Design review of the part built by this model. Coordinates are the model's own, in mm. A direction names the side the tool comes from. Give positions to 0.01 mm unless a question says otherwise; leave off trailing zeros. Write each loop counter-clockwise with the first axis right and the second up, starting at its lowest first coordinate (ties: lowest second). Pieces come first, ordered by that corner, then holes. Notation, with made-up numbers: M -15.75,72 L 39.25,72 A24 ccw 39.25,99 Z; hole C 71,27.25 d10. An arc over 180 degrees is marked long. One line per item, written item: value. Start each with the question number.
```python
from build123d import *

# Parameters (mm, degrees)
BOSS_EXTRUDE1_DEPTH = 10
CHAMFER1_SIZE       = 0.4


with BuildPart() as part:
    # Sketch1 → Boss-Extrude1 (new body)
    with BuildSketch(Plane(origin=(0, 0, 0), x_dir=(1, 0, 0), z_dir=(0, 1, 0))):
        with BuildLine():
            Line((0, 0.4), (7, 0.4))
            ThreePointArc((7, 0.4), (7.282842712, 0.517157288), (7.4, 0.8))
            Line((7.4, 0.8), (7.4, 2.4))
            ThreePointArc((7.4, 2.4), (7.282842712, 2.682842712), (7, 2.8))
            Line((7, 2.8), (-4, 2.8))
            ThreePointArc((-4, 2.8), (-4.282842712, 2.682842712), (-4.4, 2.4))
            Line((-4.4, 2.4), (-4.4, -8.3))
            ThreePointArc((-4.4, -8.3), (-4.282842712, -8.582842712), (-4, -8.7))
            Line((-4, -8.7), (7, -8.7))
            ThreePointArc((7, -8.7), (7.282842712, -8.582842712), (7.4, -8.3))
            Line((7.4, -8.3), (7.4, -0.8))
            ThreePointArc((7.4, -0.8), (7.282842712, -0.517157288), (7, -0.4))
            Line((7, -0.4), (0, -0.4))
            ThreePointArc((0, -0.4), (-0.4, 0), (0, 0.4))
        make_face()
    extrude(amount=BOSS_EXTRUDE1_DEPTH)

    # Chamfer1
    chamfer1_edges = [part.edges().sort_by_distance(p)[0] for p in [
        (7.282842712, 10, -0.517157288),
        (3.5, 0, 0.4),
        (7.282842712, 0, 0.517157288),
        (7.4, 0, 4.55),
        (7.282842712, 0, 8.582842712),
        (1.5, 0, 8.7),
        (-4.282842712, 0, 8.582842712),
        (-4.4, 0, 2.95),
        (-4.282842712, 0, -2.682842712),
        (7.4, 10, -1.6),
        (1.5, 0, -2.8),
        (7.282842712, 0, -2.682842712),
        (7.4, 0, -1.6),
        (7.282842712, 0, -0.517157288),
        (3.5, 0, -0.4),
        (-0.4, 0, 0),
        (7.282842712, 10, -2.682842712),
        (1.5, 10, -2.8),
        (-4.282842712, 10, -2.682842712),
        (-4.4, 10, 2.95),
        (-4.282842712, 10, 8.582842712),
        (1.5, 10, 8.7),
        (7.282842712, 10, 8.582842712),
        (7.4, 10, 4.55),
        (-0.4, 10, 0),
        (7.282842712, 10, 0.517157288),
        (3.5, 10, 0.4),
        (3.5, 10, -0.4),
    ]]
    chamfer(chamfer1_edges, length=CHAMFER1_SIZE - 0.0001)  # a hair under: the kernel refuses the full size


solid = part.part
```
Q1. Take a section at A-A, the plane x = 1.5. Give the boundary of the cut face in (y, z).
Q2. The part is to be moulded in two halves that separate along Z. For faces 3 (the face through (-4.4, 5, 3)), 4 (the face through (1, 5, 8.7)), 5 (the face through (2, 5, -2.8)), 6 (the face through (-0.4, 4.9, 0)), say which applies: pulls with the +Z half, pulls with the -Z half, needs draft (parallel to the pull), parting line crosses it, or undercut.
Q3. Take a section at B-B, the plane y = 5.75. Give the boundary of the cut face in (x, z).
Q4. Take a section at C-C, the plane z = 0. Give the boundary of the cut face in (x, y).
Q5. Machinability: for faces 1 (the face through (1, 0, 3)), 2 (the face through (4, 5, 0.4)), which of the approach directions +Z, -Z, +X, -X, +Y, -Y give a long, thin tool a straight path to every point of the face, cutting with its end or side? Answer none if there is none.
Q6. Wall thickness on line 1 (Z direction, x = 2, y = 4); line 2 (Z direction, x = -2, y = 9.75): over which ranges is each line inside the solid? List them lowest first. Write a range as from..to.
Results list:
1. outline: M 0,-2.4 L 0.4,-2.8 L 9.6,-2.8 L 10,-2.4 L 10,-0.8 L 9.6,-0.4 L 0.4,-0.4 L 0,-0.8 Z; M 0,0.8 L 0.4,0.4 L 9.6,0.4 L 10,0.8 L 10,8.3 L 9.6,8.7 L 0.4,8.7 L 0,8.3 Z
2. face 3: needs draft
2. face 4: pulls with the +Z half
2. face 5: pulls with the -Z half
2. face 6: undercut
3. outline: M -4.4,-2.4 A0.4 ccw -4,-2.8 L 7,-2.8 A0.4 ccw 7.4,-2.4 L 7.4,-0.8 A0.4 ccw 7,-0.4 L 0,-0.4 A0.4 cw 0,0.4 L 7,0.4 A0.4 ccw 7.4,0.8 L 7.4,8.3 A0.4 ccw 7,8.7 L -4,8.7 A0.4 ccw -4.4,8.3 Z
4. outline: M -4.4,0.4 L -4,0 L -0.8,0 L -0.4,0.4 L -0.4,9.6 L -0.8,10 L -4,10 L -4.4,9.6 Z
5. face 1: +Z, -Z, +X, -X, -Y
5. face 2: +X, +Y, -Y
6. line 1: z = -2.8..-0.4, 0.4..8.7
6. line 2: z = -2.65..8.55
